The figure shows three views and two pictorial views of one solid part (mm, origin at its lowest corner). Answer the questions. A direction names the side the tool comes from. Give positions to 0.01 mm unless a question says otherwise; leave off trailing zeros. Order: outer loops, then holes, each group sorted by start corner. A loop starts at its lowest first (then second) coordinate and runs counter-clockwise, first axis right, second up. Notation, with made-up numbers: (56.5, 44) - (83.5, 44) arc R24 ccw to (83.5, 81) - close; hole circle Ø5 at (-13.5, 25). An arc over 180 degrees is marked (long way). Use a Markdown table: item, result. Add a question column.
1. A cutting plane is placed at A-A on x = 7.62. Determine the outline of the cut face in (y, z).
2. Consider L1, parallel to Z at x = 7.62, y = 4.1; L2, parallel to Y at x = 43.2, z = 8.89; L3, parallel to Z at x = 44, y = 63. Determine where each line is inside the solid, lowest interval first.
3. A cutting plane is placed at C-C on y = 30. Determine the outline of the cut face in (x, z).
4. Which of the six approach directions +Z, -Z, +X, -X, +Y, -Y give full straight-line access (tool end or side, diameter ignored) to the marked faces 1 and 2?
5. A cutting plane is placed at B-B on z = 8.89. Determine the outline of the cut face in (x, y), and give its area (3 significant figures).
6. Flat-ended cylindrical pins translate along their axes: P1, Ø1, axis at y = 48, z = 66.5, coming from the -X side; P2, Ø5, axis at x = 22, z = 76, coming from the +Y side; P3, Ø3, axis at x = 7.62, z = 26.67, coming from the -Y side. Find the tip coordinate at first contact, or state that the pin passes through.
7. A cutting plane is placed at D-D on z = 88.5. Determine the outline of the cut face in (x, y).
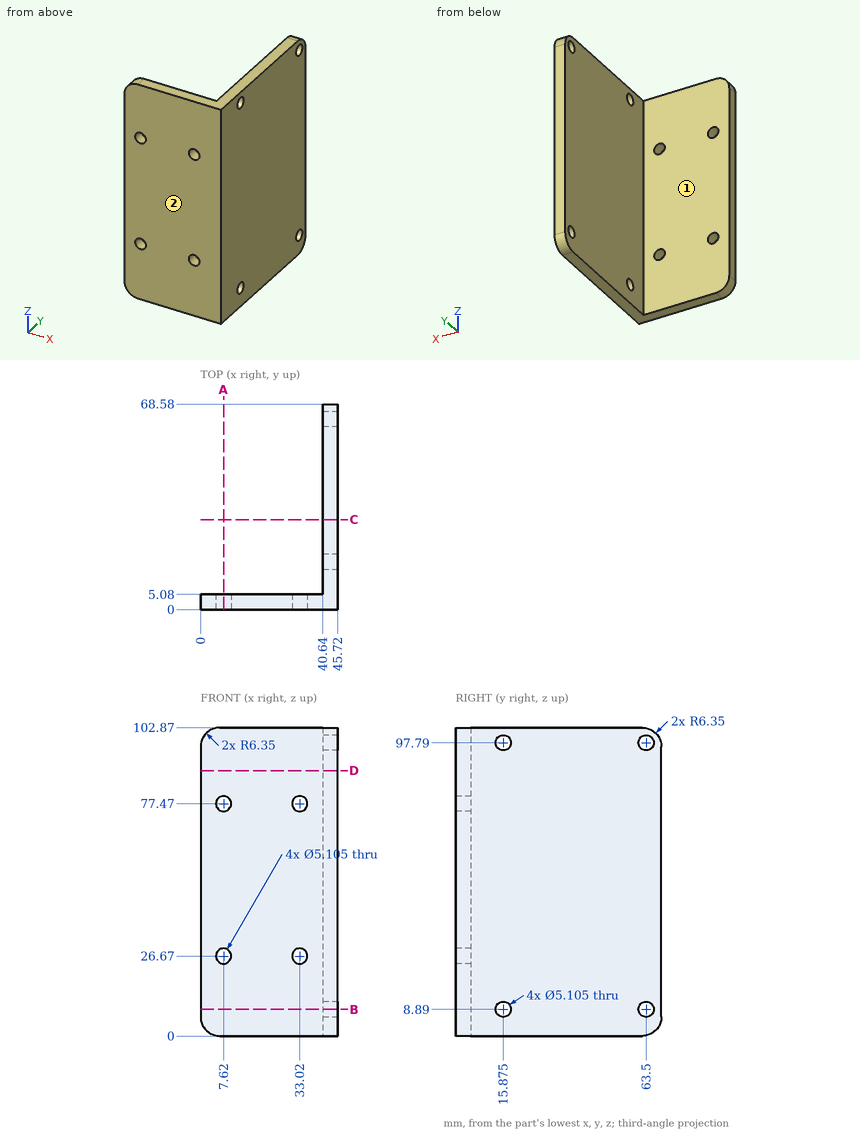
Output values:
| question | item | result |
|---|---|---|
| 1 | outline | (0, 0) - (5.08, 0) - (5.08, 24.12) - (0, 24.12) - close; (0, 29.22) - (5.08, 29.22) - (5.08, 74.92) - (0, 74.92) - close; (0, 80.02) - (5.08, 80.02) - (5.08, 102.87) - (0, 102.87) - close |
| 2 | L1 | 0 to 24.12, 29.22 to 74.92, 80.02 to 102.87 |
| 2 | L2 | 0 to 13.32, 18.43 to 60.95, 66.05 to 68.58 |
| 2 | L3 | 0.05 to 6.39, 11.39 to 95.29, 100.29 to 102.82 |
| 3 | outline | (40.64, 0) - (45.72, 0) - (45.72, 102.87) - (40.64, 102.87) - close |
| 4 | face 1 | +Z, -Z, -X, +Y |
| 4 | face 2 | +Z, -Z, +X, -X, -Y |
| 5 | outline | (0, 0) - (45.72, 0) - (45.72, 13.32) - (40.64, 13.32) - (40.64, 5.08) - (0, 5.08) - close; (40.64, 18.43) - (45.72, 18.43) - (45.72, 60.95) - (40.64, 60.95) - close; (40.64, 66.05) - (45.72, 66.05) - (45.72, 68.58) - (40.64, 68.58) - close |
| 5 | area | 503 mm² |
| 6 | P1 | x = 40.64 |
| 6 | P2 | y = 5.08 |
| 6 | P3 | through |
| 7 | outline | (0, 0) - (45.72, 0) - (45.72, 68.58) - (40.64, 68.58) - (40.64, 5.08) - (0, 5.08) - close |
